For this review, take the finished solid that the model builds, in its own axes (mm). Round coordinates to 2 decimals unless told otherwise and drop trailing zeros. Write each loop counter-clockwise with the first axis right and the second up, starting at its lowest first coordinate (ties: lowest second). Pieces come first, ordered by that corner, then holes. Notation, with made-up numbers: (55, -23.75) -> (75, -23.75) arc R16 ccw to (75, 4.25) -> close; hole circle Ø7 at (6.5, 56.5). An arc over 180 degrees is marked (long way). Answer as CSV lines item,"result". Start each with the question number.
Item 1: For pin 1 Ø6 at (x, z) = (-64.5, -8.5) entering from +Y; pin 2 Ø4 at (x, z) = (-73.5, -11) entering from +Y; pin 3 Ø8 at (y, z) = (-100, -12.5) entering from +X, all flat-tipped, find the tip position at first contact; note any pin that passes through.
Item 2: Wall thickness on probe 1 along X at (y, z) = (-73, 0.25); probe 2 along Z at (x, y) = (-37, -79.5); probe 3 along X at (y, z) = (-97.5, -14.25): over which ranges is each line inside the solid? List them lowest first. Write a range as from..to.
Item 3: Take a section at A-A on x = -27. Give the boundary of the cut face in (y, z), then the cut area to 3 significant figures.
Item 4: Take a section at B-B on z = 1.5. Give the boundary of the cut face in (x, y).
```python
from build123d import *

# Parameters (mm, degrees)
THREE_MILLIMETRE_STRUT_CORE_SKETCH_R = 1.5
THREE_MILLIMETRE_STRUT_CORE_DEPTH    = 64.364941753


with BuildPart() as part:
    # Three millimetre strut core sketch → Three millimetre strut core (new body)
    with BuildSketch(Plane(origin=(-47.508082523, -23.76220438, -12.729752346), x_dir=(-0.20842845999452628, -0.10425004340144392, 0.9724656834640013), z_dir=(-0.8697399638531149, -0.435019425763827, -0.23304612093938143))):
        with Locations(Location((13.090181548, -53.527480937, 0), (0, 0, 270))):
            Circle(THREE_MILLIMETRE_STRUT_CORE_SKETCH_R)
    extrude(amount=THREE_MILLIMETRE_STRUT_CORE_DEPTH)

    # Ball end 1 profile → Ball end 1 (revolve)
    with BuildSketch(Plane(origin=(0, -73, 0), x_dir=(-1, 0, 0), z_dir=(0, -1, 0))):
        with BuildLine():
            Line((26.291651246, -3), (26.291651246, 3))
            ThreePointArc((26.291651246, 3), (23.291651246, 0), (26.291651246, -3))
        make_face()
    revolve(axis=Axis((-26.291651246, -73, -10), (0, 0, 1)))

    # Ball end 2 profile → Ball end 2 (revolve)
    with BuildSketch(Plane(origin=(0, -101.000000001, 0), x_dir=(-1, 0, 0), z_dir=(0, -1, 0))):
        with BuildLine():
            Line((82.272413359, 12), (82.272413359, 18))
            ThreePointArc((82.272413359, 18), (79.272413359, 15), (82.272413359, 12))
        make_face()
    revolve(axis=Axis((-82.272413359, -101.000000001, -25), (0, 0, 1)))


solid = part.part
```
Output values:
1,pin 1,"stops at y = -88.97"
1,pin 2,"stops at y = -94.02"
1,pin 3,"stops at x = -69.06"
2,probe 1,"x = -29.28..-23.3"
2,probe 2,"z = -4.12..-1.86"
2,probe 3,"x = -78.49..-73.93"
3,outline,"circle Ø5.83 at (-73, 0)"
3,area,"26.7 mm^2"
4,outline,"circle Ø5.2 at (-26.29, -73)"
